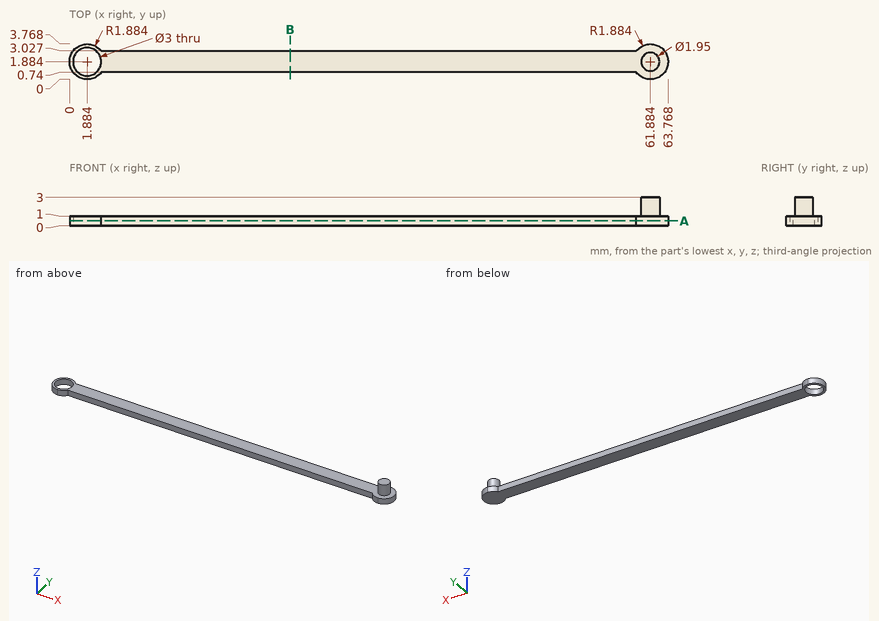
Design review of the part shown in the three views and the two pictorial views. Dimensions are in mm from the part's minimum x, y and z. Round coordinates to 2 decimals unless told otherwise and drop trailing zeros. Loops run counter-clockwise (first coordinate to the right, second up) from the corner with the lowest first, then second, coordinate; pieces in that order, holes last. Notation, with made-up numbers: (21, 63) -> (28, 63) arc R3 cw to (28, 67) -> close; hole circle Ø7 at (-9, -12.5). An arc over 180 degrees is marked (long way). Return JSON: item names as keys, results as strings.
(1) For line 1 (X direction, y = 1.7, z = 0.3) (1 decimal); line 2 (Z direction, x = 15.5, y = 1.8); line 3 (X direction, y = 1.8, z = 1.9) (1 decimal), list the stretches that pass through material, from the lowest coordinate up.
Solved:
{"line 1": "0 to 0.4, 3.4 to 63.8", "line 2": "0 to 1", "line 3": "60.9 to 62.9"}
(2) Add section B-B on x = 23.5. Write out the cut boundary in (y, z).
Solved:
{"outline": "(0.74, 0) -> (3.03, 0) -> (3.03, 1) -> (0.74, 1) -> close"}
(3) Add section A-A on z = 0.5. Write out the cut boundary in (x, y).
Solved:
{"outline": "(3.38, 0.74) -> (60.39, 0.74) arc R1.88 ccw (long way) to (60.39, 3.03) -> (3.38, 3.03) arc R1.88 ccw (long way) to start; hole circle Ø3 at (1.88, 1.88)"}
(4) For pin 1 (1.5 mm diameter, centred on x = 10.5, y = 1.5, fed in from +Z); pin 2 (1.5 mm diameter, centred on y = 0.5, z = 2, fed in from +X) (1 decimal), all flat-tipped, find the tip position at first contact; note any pin that passes through.
Solved:
{"pin 1": "z = 1", "pin 2": "x = 62.6"}
